Source: three-view drawing plus pictorial views. Frame: mm from the lowest corner of the part. A direction names the side the tool comes from. Give positions to 0.01 mm unless a question says otherwise; leave off trailing zeros. Order: outer loops, then holes, each group sorted by start corner. A loop starts at its lowest first (then second) coordinate and runs counter-clockwise, first axis right, second up.
1) Material intervals for line 1 (Z direction, x = 4.75, y = 12.5); line 2 (X direction, y = 12.25, z = 3.75); line 3 (Z direction, x = 7.75, y = 11.5), sorted ascending.
2) First-contact query: P1, Ø6, axis at x = 2.5, z = 4.5, coming from the +Y side; P2, Ø1, axis at y = 7.5, z = 2.5, coming from the -X side; P3, Ø1, axis at x = 3.5, z = 1.5, coming from the -Y side; P4, Ø4, axis at x = 10, y = 6.5, coming from the +Z side. Flat tips, straight axial feed; report the tip coordinate or a pass-through.
3) Section D-D, the plane z = 0.5. Return loops of the section in (x, y).
4) Section C-C, the plane y = 4.5. Return loops of the section in (x, z).
5) Section B-B, the plane x = 5. Return loops of the section in (y, z), plus the area to 3 significant figures.
6) Draft query along Z for the marked faces 3, 4, 5 and 6. Return one class per face: released by +Z, released by -Z, zero draft, split by the parting line, or undercut.
7) Section A-A, the plane y = 10.5. Return loops of the section in (x, z), plus the area to 3 significant figures.
8) Access query for the marked faces 1 and 2. Directions: +Z, -Z, +X, -X, +Y, -Y. A direction counts if a zero-diameter tool reaches every point of the face in a straight line with its end or side. Return the directions, or none.
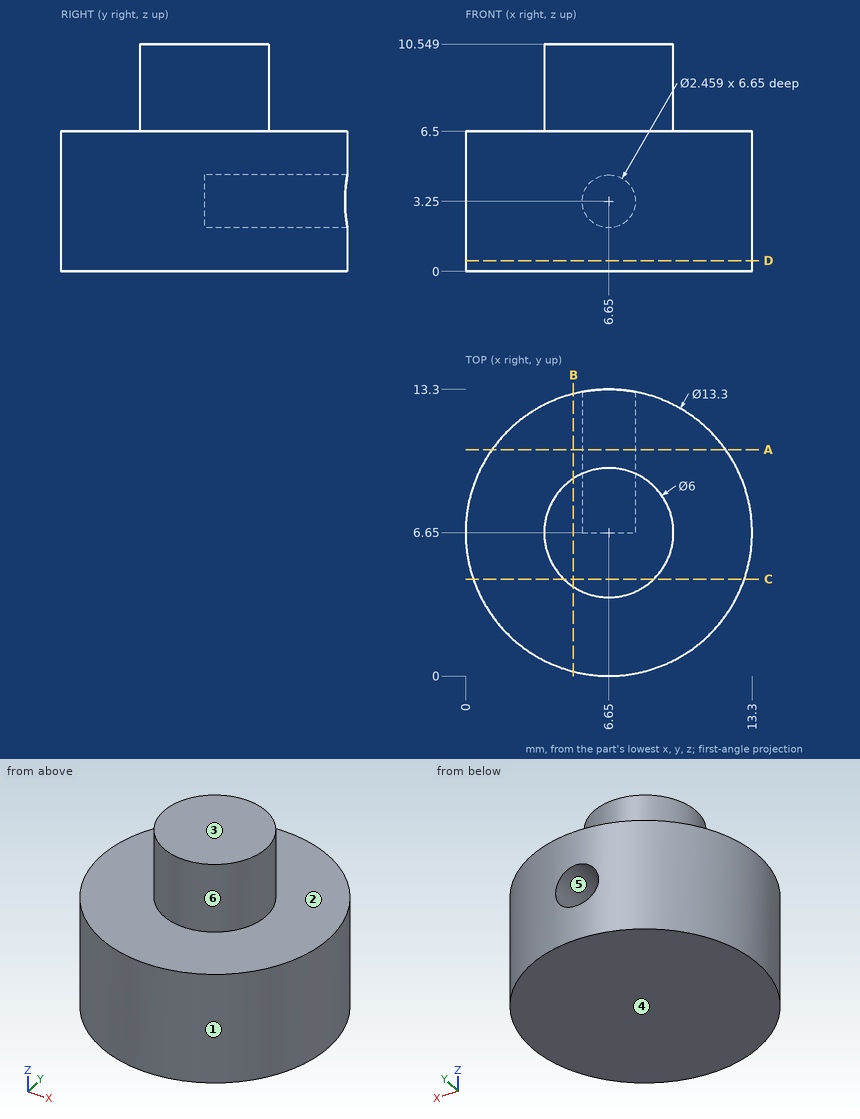
From the geometry:
1. line 1: z = 0 to 6.5
1. line 2: x = 3.06 to 5.53, 7.77 to 10.24
1. line 3: z = 0 to 2.7, 3.8 to 6.5
2. P1: stops at y = 13.2
2. P2: stops at x = 0.01
2. P3: stops at y = 0.55
2. P4: stops at z = 10.55
3. outline: circle Ø13.3 at (6.65, 6.65)
4. outline: (0.36, 0) - (12.94, 0) - (12.94, 6.5) - (8.74, 6.5) - (8.74, 10.55) - (4.56, 10.55) - (4.56, 6.5) - (0.36, 6.5) - close
5. outline: (0.21, 0) - (13.09, 0) - (13.09, 6.5) - (9.16, 6.5) - (9.16, 10.55) - (4.14, 10.55) - (4.14, 6.5) - (0.21, 6.5) - close
5. area: 104 mm2
6. face 3: released by +Z
6. face 4: released by -Z
6. face 5: undercut
6. face 6: zero draft
7. outline: (1.23, 0) - (12.07, 0) - (12.07, 6.5) - (1.23, 6.5) - close; hole circle Ø2.46 at (6.65, 3.25)
7. area: 65.7 mm2
8. face 1: +Z, -Z
8. face 2: +Z
